from build123d import *

# Parameters (mm, degrees)
SKETCH1_W           = 250
SKETCH1_H           = 150
SKETCH1_R           = 1.5
SKETCH1_R_2         = 10
SKETCH1_RX          = 5.5
SKETCH1_RY          = 3.5
BOSS_EXTRUDE3_DEPTH = 4


with BuildPart() as part:
    # Sketch1 → Boss-Extrude3 (new body)
    with BuildSketch(Plane.XY):
        with Locations((64.901502586, -41.133333333)):
            Rectangle(SKETCH1_W, SKETCH1_H)
        with Locations((-32.098497414, -92.133333333)):
            Circle(SKETCH1_R, mode=Mode.SUBTRACT)
        with Locations((-17.098497414, -92.133333333)):
            Circle(SKETCH1_R, mode=Mode.SUBTRACT)
        with Locations((-32.098497414, -107.133333333)):
            Circle(SKETCH1_R, mode=Mode.SUBTRACT)
        with Locations((-47.098497414, -92.133333333)):
            Circle(SKETCH1_R, mode=Mode.SUBTRACT)
        with Locations((-32.098497414, -77.133333333)):
            Circle(SKETCH1_R, mode=Mode.SUBTRACT)
        with Locations((176.901502586, -92.133333333)):
            Circle(SKETCH1_R, mode=Mode.SUBTRACT)
        with Locations((161.901502586, -92.133333333)):
            Circle(SKETCH1_R, mode=Mode.SUBTRACT)
        with Locations((161.901502586, -77.133333333)):
            Circle(SKETCH1_R, mode=Mode.SUBTRACT)
        with Locations((146.901502586, -92.133333333)):
            Circle(SKETCH1_R, mode=Mode.SUBTRACT)
        with Locations((161.901502586, -107.133333333)):
            Circle(SKETCH1_R, mode=Mode.SUBTRACT)
        with Locations((176.901502586, 9.866666667)):
            Circle(SKETCH1_R, mode=Mode.SUBTRACT)
        with Locations((161.901502586, 9.866666667)):
            Circle(SKETCH1_R, mode=Mode.SUBTRACT)
        with Locations((161.901502586, 24.866666667)):
            Circle(SKETCH1_R, mode=Mode.SUBTRACT)
        with Locations((146.901502586, 9.866666667)):
            Circle(SKETCH1_R, mode=Mode.SUBTRACT)
        with Locations((161.901502586, -5.133333333)):
            Circle(SKETCH1_R, mode=Mode.SUBTRACT)
        with Locations((-17.098497414, 9.866666667)):
            Circle(SKETCH1_R, mode=Mode.SUBTRACT)
        with Locations((-32.098497414, 9.866666667)):
            Circle(SKETCH1_R, mode=Mode.SUBTRACT)
        with Locations((-32.098497414, 24.866666667)):
            Circle(SKETCH1_R, mode=Mode.SUBTRACT)
        with Locations((-47.098497414, 9.866666667)):
            Circle(SKETCH1_R, mode=Mode.SUBTRACT)
        with Locations((-32.098497414, -5.133333333)):
            Circle(SKETCH1_R, mode=Mode.SUBTRACT)
        with Locations((-32.098497414, -41.133333333)):
            Circle(SKETCH1_R, mode=Mode.SUBTRACT)
        with Locations((161.901502586, -41.133333333)):
            Circle(SKETCH1_R, mode=Mode.SUBTRACT)
        with Locations((64.901502586, 9.866666667)):
            Circle(SKETCH1_R, mode=Mode.SUBTRACT)
        with Locations((64.901502586, -92.133333333)):
            Circle(SKETCH1_R, mode=Mode.SUBTRACT)
        with Locations((94.901502586, -26.133333333)):
            Circle(SKETCH1_R_2, mode=Mode.SUBTRACT)
        with Locations((94.901502586, -56.133333333)):
            Circle(SKETCH1_R_2, mode=Mode.SUBTRACT)
        with Locations((-46.598497414, -41.133333333)):
            Ellipse(SKETCH1_RX, SKETCH1_RY, mode=Mode.SUBTRACT)
        with Locations(Location((9.901502586, 15.366666667), (0, 0, -90))):
            Ellipse(SKETCH1_RX, SKETCH1_RY, mode=Mode.SUBTRACT)
        with Locations(Location((66.401502586, -42.699426362), (0, 0, 180))):
            Ellipse(SKETCH1_RX, SKETCH1_RY, mode=Mode.SUBTRACT)
        with Locations(Location((8.835409557, -96.133333333), (0, 0, -90))):
            Ellipse(SKETCH1_RX, SKETCH1_RY, mode=Mode.SUBTRACT)
    extrude(amount=BOSS_EXTRUDE3_DEPTH)


solid = part.part
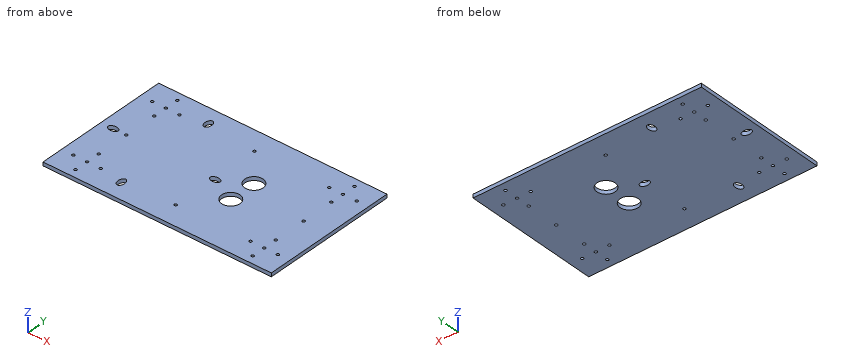
The model under review builds one solid part; all positions refer to its coordinate system, in mm. Give positions to 0.01 mm unless a question says otherwise; leave off trailing zeros. Order: outer loops, then holes, each group sorted by start corner. A loop starts at its lowest first (then second) coordinate and runs counter-clockwise, first axis right, second up. Notation, with made-up numbers: M -11.5,82.5 L 23.5,82.5 A17 ccw 23.5,87.5 Z; hole C 87.25,81 d8. An arc over 180 degrees is marked long. Use one line per item in the form item = value. Start each with the question number.
Item 1: We need section A-A on y = -22.5. Give the boundary of the cut face in (x, z).
Item 2: To check wall thickness, follow line 1 along Y through (x, z) = (-47, 1.5); line 2 along X through (y, z) = (16, 0.3); line 3 along X through (y, z) = (-41, 3). State the ranges of each line that lie inside material, in increasing order. Write a range as from..to.
Item 3: Insertion check: pin 1 Ø2 at (x, y) = (130, -0.5) entering from -Z; pin 2 Ø1.8 at (x, y) = (176.9, -92.13) entering from +Z (1 decimal). Each pin has a flat end and moves straight along its axis. Give the tip position at first contact, or say it passes through.
Item 4: We need section B-B on z = 0.95. Give the number of separate pieces and of enclosed holes in the cut face, plus the area to 3 significant figures.
Completed:
q1.outline = M -60.1,0 L 85.58,0 L 85.58,4 L -60.1,4 Z; M 104.22,0 L 189.9,0 L 189.9,4 L 104.22,4 Z
q2.line_1 = -116.13..-93.63, -90.64..-44.62, -37.64..8.37, 11.36..33.87
q2.line_2 = -60.1..6.42, 13.38..189.9
q2.line_3 = -60.1..-52.09, -41.1..-33.59, -30.6..61.59, 71.21..160.41, 163.4..189.9
q3.pin_1 = 0
q3.pin_2 = through
q4.separate_pieces = 1
q4.enclosed_holes = 30
q4.area = 36,500 mm²
